Autodesk Fusion 360 part; units mm, degrees
sketch "草图1" plane through (0, 0, 0) normal (0, 1, 0) x (1, 0, 0)
  line L0 (0, 0) -> (95.2, 0)
  line L1 (95.2, 0) -> (95.2, 95.4)
  line L2 (95.2, 95.4) -> (0, 95.4)
  line L3 (0, 95.4) -> (0, 0)
  line L4 (-1.5, 96.9) -> (96.7, 96.9)
  line L5 (96.7, 96.9) -> (96.7, -1.5)
  line L6 (96.7, -1.5) -> (-1.5, -1.5)
  line L7 (-1.5, -1.5) -> (-1.5, 96.9)
  line L8 (-2.5, 97.9) -> (97.7, 97.9)
  line L9 (97.7, 97.9) -> (97.7, -2.5)
  line L10 (97.7, -2.5) -> (-2.5, -2.5)
  line L11 (-2.5, -2.5) -> (-2.5, 97.9)
  line L12 (-4.5, 100.9) -> (99.7, 100.9)
  line L13 (99.7, 100.9) -> (99.7, -5.5)
  line L14 (99.7, -5.5) -> (-4.5, -5.5)
  line L15 (-4.5, -5.5) -> (-4.5, 100.9)
  line L16 (99.7, 100.9) -> (79.7, 100.9)
  line L17 (79.7, 100.9) -> (79.7, 80.9)
  line L18 (79.7, 80.9) -> (99.7, 80.9)
  line L19 (99.7, 80.9) -> (99.7, 100.9)
  line L20 (79.7, 100.9) -> (99.7, 80.9)
  dimension "d1" = 95.2
  dimension "d2" = 95.4
  dimension "d3" = 1.5
  dimension "d4" = 1.5
  dimension "d5" = 1.5
  dimension "d6" = 1.5
  dimension "d7" = 1
  dimension "d8" = 1
  dimension "d9" = 1
  dimension "d10" = 1
  dimension "d11" = 3
  dimension "d12" = 2
  dimension "d13" = 2
  dimension "d14" = 3
  dimension "d21" = 20
  dimension "d22" = 20
extrude "拉伸1" add sketch "草图1" along normal blind 2 contours L0 L1 L2 L3 L17 L18 | L0 L1 L2 L3 L4 L5 L6 L7 L17 L18 | L1 L2 L17 L18 L20 | L1 L5 L18 L20 | L2 L4 L17 L20 | L1 L2 L20 | L1 L2 L4 L5 L20 | L4 L5 L6 L7 L8 L9 L10 L11 L17 L18 | L5 L9 L18 L20 | L4 L8 L17 L20 | L4 L5 L8 L9 L20
extrude "拉伸2" add sketch "草图1" along normal blind 22 contours L8 L9 L10 L11 L12 L13 L14 L15 L17 L18 | L9 L18 L20 | L8 L17 L20 | L8 L9 L12 L13 L16 L19 L20
fillet "圆角1" radius 5 4 edges at (-4.5, 11, 5.5) (99.7, 11, 5.5) (-4.5, 11, -100.9) (99.7, 11, -100.9)
extrude "拉伸3" [suppressed]
fillet "圆角2" [suppressed]
sketch "草图2" plane through (0, 2, 0) normal (0, 1, 0) x (-1, 0, 0)
  line L0 (-97.7, -97.9) -> (2.5, -97.9)
  line L1 (2.5, -97.9) -> (2.5, 2.5)
  line L2 (2.5, 2.5) -> (-97.7, 2.5)
  line L3 (-97.7, 2.5) -> (-97.7, -97.9)
  line L4 (2.5, 2.5) -> (2.5, -20)
  line L5 (2.5, -20) -> (-5.5, -20)
  line L6 (-5.5, -20) -> (-5.5, -22)
  line L7 (-5.5, -22) -> (2.5, -22)
  line L8 (2.5, -22) -> (2.5, -20)
  line L9 (-5.5, -20) -> (-3.5, -20)
  line L10 (-3.5, -20) -> (-3.5, 2.5)
  line L11 (-3.5, 2.5) -> (-5.5, 2.5)
  line L12 (-5.5, 2.5) -> (-5.5, -20)
  line L13 (-97.7, 2.5) -> (-91.7, 2.5)
  line L14 (-91.7, 2.5) -> (-91.7, -20)
  line L15 (-91.7, -20) -> (-97.7, -20)
  line L16 (-97.7, -20) -> (-97.7, 2.5)
  line L17 (-97.7, -20) -> (-89.7, -20)
  line L18 (-89.7, -20) -> (-89.7, -23)
  line L19 (-89.7, -23) -> (-97.7, -23)
  line L20 (-97.7, -23) -> (-97.7, -20)
  line L21 (-89.7, -20) -> (-91.7, -20)
  line L22 (-91.7, -20) -> (-91.7, 2.5)
  line L23 (-91.7, 2.5) -> (-89.7, 2.5)
  line L24 (-89.7, 2.5) -> (-89.7, -20)
  line L25 (-91.7, -97.9) -> (-91.7, -75.4)
  line L26 (-91.7, -97.9) -> (-97.7, -97.9)
  line L27 (-97.7, -97.9) -> (-97.7, -75.4)
  line L28 (-97.7, -75.4) -> (-91.7, -75.4)
  line L29 (2.5, -97.9) -> (2.5, -75.4)
  line L30 (-3.5, -75.4) -> (2.5, -75.4)
  line L31 (-3.5, -97.9) -> (-3.5, -75.4)
  line L32 (2.5, -97.9) -> (-3.5, -97.9)
  line L33 (2.5, -75.4) -> (-5.5, -75.4)
  line L34 (-5.5, -75.4) -> (-5.5, -73.4)
  line L35 (-5.5, -73.4) -> (2.5, -73.4)
  line L36 (2.5, -73.4) -> (2.5, -75.4)
  line L37 (-5.5, -75.4) -> (-3.5, -75.4)
  line L38 (-3.5, -75.4) -> (-3.5, -97.9)
  line L39 (-3.5, -97.9) -> (-5.5, -97.9)
  line L40 (-5.5, -97.9) -> (-5.5, -75.4)
  line L41 (-97.7, -75.4) -> (-89.7, -75.4)
  line L42 (-89.7, -75.4) -> (-89.7, -73.4)
  line L43 (-89.7, -73.4) -> (-97.7, -73.4)
  line L44 (-97.7, -73.4) -> (-97.7, -75.4)
  line L45 (-89.7, -75.4) -> (-91.7, -75.4)
  line L46 (-91.7, -75.4) -> (-91.7, -97.9)
  line L47 (-91.7, -97.9) -> (-89.7, -97.9)
  line L48 (-89.7, -97.9) -> (-89.7, -75.4)
  line L49 (-47.6, -97.9) -> (-47.6, -91.9)
  line L50 (-47.6, -91.9) -> (-36.35, -91.9)
  line L51 (-47.6, -91.9) -> (-58.85, -91.9)
  line L52 (-36.35, -91.9) -> (-58.85, -91.9)
  line L53 (-58.85, -91.9) -> (-58.85, -97.9)
  line L54 (-58.85, -97.9) -> (-36.35, -97.9)
  line L55 (-36.35, -97.9) -> (-36.35, -91.9)
  line L56 (-47.6, 2.5) -> (-36.35, 2.5)
  line L57 (-36.35, -3.5) -> (-36.35, 2.5)
  line L58 (-58.85, -3.5) -> (-36.35, -3.5)
  line L59 (-36.35, 2.5) -> (-58.85, 2.5)
  line L60 (-58.85, 2.5) -> (-58.85, -3.5)
  line L61 (-36.35, -97.9) -> (-34.35, -97.9)
  line L62 (-34.35, -97.9) -> (-34.35, -89.9)
  line L63 (-34.35, -89.9) -> (-36.35, -89.9)
  line L64 (-36.35, -89.9) -> (-36.35, -97.9)
  line L65 (-36.35, -89.9) -> (-58.85, -89.9)
  line L66 (-58.85, -89.9) -> (-58.85, -91.9)
  line L67 (-58.85, -91.9) -> (-36.35, -91.9)
  line L68 (-36.35, -91.9) -> (-36.35, -89.9)
  line L69 (-58.85, -89.9) -> (-60.85, -89.9)
  line L70 (-60.85, -89.9) -> (-60.85, -97.9)
  line L71 (-60.85, -97.9) -> (-58.85, -97.9)
  line L72 (-58.85, -97.9) -> (-58.85, -89.9)
  line L73 (-36.35, 2.5) -> (-34.35, 2.5)
  line L74 (-34.35, 2.5) -> (-34.35, -5.5)
  line L75 (-34.35, -5.5) -> (-36.35, -5.5)
  line L76 (-36.35, -5.5) -> (-36.35, 2.5)
  line L77 (-58.85, 2.5) -> (-60.85, 2.5)
  line L78 (-60.85, 2.5) -> (-60.85, -5.5)
  line L79 (-60.85, -5.5) -> (-58.85, -5.5)
  line L80 (-58.85, -5.5) -> (-58.85, 2.5)
  line L81 (-36.35, -5.5) -> (-58.85, -5.5)
  line L82 (-58.85, -5.5) -> (-58.85, -3.5)
  line L83 (-58.85, -3.5) -> (-36.35, -3.5)
  line L84 (-36.35, -3.5) -> (-36.35, -5.5)
  dimension "d27" = 22.5
  dimension "d28" = 8
  dimension "d29" = 2
  dimension "d32" = 6
  dimension "d33" = 22.5
  dimension "d34" = 8
  dimension "d35" = 3
  dimension "d38" = 77.9
  dimension "d39" = 0
  dimension "d42" = 94.2
  dimension "d43" = 0
  dimension "d44" = 8
  dimension "d45" = 2
  dimension "d46" = 8
  dimension "d47" = 2
  dimension "d50" = 6
  dimension "d51" = 11.25
  dimension "d52" = 11.25
  dimension "d55" = 0
  dimension "d56" = 94.4
  dimension "d57" = 2
  dimension "d58" = 8
  dimension "d59" = 2
  dimension "d60" = 8
  dimension "d61" = 2
  dimension "d62" = 8
  dimension "d63" = 2
  dimension "d64" = 8
extrude "拉伸4" [suppressed]
extrude "拉伸5" [suppressed]
extrude "拉伸6" [suppressed]
sketch "草图3" plane through (0, 2, 0) normal (0, 1, 0) x (-1, 0, 0)
  line L0 (2.5, 2.5) -> (-97.7, 2.5)
  line L1 (-97.7, 2.5) -> (-97.7, -97.9)
  line L2 (-97.7, -97.9) -> (2.5, -97.9)
  line L3 (2.5, -97.9) -> (2.5, 2.5)
  line L4 (2.5, 2.5) -> (-20, 2.5)
  line L5 (-20, 2.5) -> (-20, -4)
  line L6 (-20, -4) -> (2.5, -4)
  line L7 (2.5, -4) -> (2.5, 2.5)
  line L8 (2.5, -4) -> (-20, -4)
  line L9 (-20, -4) -> (-20, -6)
  line L10 (-20, -6) -> (2.5, -6)
  line L11 (2.5, -6) -> (2.5, -4)
  line L12 (-20, -6) -> (-22, -6)
  line L13 (-22, -6) -> (-22, 2.5)
  line L14 (-22, 2.5) -> (-20, 2.5)
  line L15 (-20, 2.5) -> (-20, -6)
  line L16 (-20, -91.4) -> (-20, -97.9)
  line L17 (-20, -97.9) -> (2.5, -97.9)
  line L18 (2.5, -97.9) -> (2.5, -91.4)
  line L19 (2.5, -91.4) -> (-20, -91.4)
  line L20 (2.5, -97.9) -> (-20, -97.9)
  line L21 (2.5, -91.4) -> (-20, -91.4)
  line L22 (-20, -91.4) -> (-20, -89.4)
  line L23 (-20, -89.4) -> (2.5, -89.4)
  line L24 (2.5, -89.4) -> (2.5, -91.4)
  line L25 (-20, -89.4) -> (-22, -89.4)
  line L26 (-22, -89.4) -> (-22, -97.9407)
  line L27 (-22, -97.9407) -> (-20, -97.9407)
  line L28 (-20, -97.9407) -> (-20, -89.4)
  line L29 (2.5, -47.7) -> (-4, -47.7)
  line L30 (-4, -47.7) -> (-4, -58.95)
  line L31 (-4, -58.95) -> (2.5, -58.95)
  line L32 (2.5, -58.95) -> (2.5, -47.7)
  line L33 (-4, -47.7) -> (2.5, -47.7)
  line L34 (2.5, -47.7) -> (2.5, -36.45)
  line L35 (2.5, -36.45) -> (-4, -36.45)
  line L36 (-4, -36.45) -> (-4, -47.7)
  line L37 (-97.7, -36.45) -> (-97.7, -47.7)
  line L38 (-91.2, -47.7) -> (-91.2, -36.45)
  line L39 (-97.7, -47.7) -> (-97.7, -58.95)
  line L40 (-91.2, -58.95) -> (-91.2, -47.7)
  line L41 (-91.2, -36.45) -> (-97.7, -36.45)
  line L42 (-91.2, -47.7) -> (-97.7, -47.7)
  line L43 (-97.7, -47.7) -> (-91.2, -47.7)
  line L44 (-97.7, -58.95) -> (-91.2, -58.95)
  line L45 (2.5, -36.45) -> (-6, -36.45)
  line L46 (-6, -36.45) -> (-6, -34.45)
  line L47 (-6, -34.45) -> (2.5, -34.45)
  line L48 (2.5, -34.45) -> (2.5, -36.45)
  line L49 (-4, -58.95) -> (-6, -58.95)
  line L50 (-6, -58.95) -> (-6, -36.45)
  line L51 (-6, -36.45) -> (-4, -36.45)
  line L52 (-4, -36.45) -> (-4, -58.95)
  line L53 (-6, -58.95) -> (2.5, -58.95)
  line L54 (2.5, -58.95) -> (2.5, -60.95)
  line L55 (2.5, -60.95) -> (-6, -60.95)
  line L56 (-6, -60.95) -> (-6, -58.95)
  line L57 (-97.7, -36.45) -> (-89.2, -36.45)
  line L58 (-89.2, -36.45) -> (-89.2, -34.45)
  line L59 (-89.2, -34.45) -> (-97.7, -34.45)
  line L60 (-97.7, -34.45) -> (-97.7, -36.45)
  line L61 (-89.2, -36.45) -> (-91.2, -36.45)
  line L62 (-91.2, -36.45) -> (-91.2, -58.95)
  line L63 (-91.2, -58.95) -> (-89.2, -58.95)
  line L64 (-89.2, -58.95) -> (-89.2, -36.45)
  line L65 (-89.2, -58.95) -> (-97.7, -58.95)
  line L66 (-97.7, -58.95) -> (-97.7, -60.95)
  line L67 (-97.7, -60.95) -> (-89.2, -60.95)
  line L68 (-89.2, -60.95) -> (-89.2, -58.95)
  line L69 (-101, -101) -> (-85, -101)
  line L70 (-85, -101) -> (-85, -85)
  line L71 (-85, -85) -> (-101, -85)
  line L72 (-101, -85) -> (-101, -101)
  line L73 (-85, -97.9) -> (-83, -97.9)
  line L74 (-83, -97.9) -> (-83, -89.4)
  line L75 (-83, -89.4) -> (-85, -89.4)
  line L76 (-85, -89.4) -> (-85, -97.9)
  line L77 (-83, -97.9) -> (-60.5, -97.9)
  line L78 (-60.5, -97.9) -> (-60.5, -91.4)
  line L79 (-60.5, -91.4) -> (-83, -91.4)
  line L80 (-83, -91.4) -> (-83, -97.9)
  line L81 (-83, -89.4) -> (-60.5, -89.4)
  line L82 (-60.5, -89.4) -> (-60.5, -91.4)
  line L83 (-60.5, -91.4) -> (-83, -91.4)
  line L84 (-83, -91.4) -> (-83, -89.4)
  line L85 (-60.5, -89.4) -> (-58.5, -89.4)
  line L86 (-58.5, -89.4) -> (-58.5, -97.9)
  line L87 (-58.5, -97.9) -> (-60.5, -97.9)
  line L88 (-60.5, -97.9) -> (-60.5, -89.4)
  line L89 (-60.5, 2.5) -> (-83, 2.5)
  line L90 (-60.5, 2.5) -> (-83, 2.5)
  line L91 (-83, -4) -> (-60.5, -4)
  line L92 (-60.5, -4) -> (-60.5, 2.5)
  line L93 (-83, 2.5) -> (-83, -4)
  line L94 (-60.5, 2.5) -> (-58.5, 2.5)
  line L95 (-58.5, 2.5) -> (-58.5, -6)
  line L96 (-58.5, -6) -> (-60.5, -6)
  line L97 (-60.5, -6) -> (-60.5, 2.5)
  line L98 (-60.5, -6) -> (-83, -6)
  line L99 (-83, -6) -> (-83, -4)
  line L100 (-83, -4) -> (-60.5, -4)
  line L101 (-60.5, -4) -> (-60.5, -6)
  line L102 (-83, -6) -> (-85, -6)
  line L103 (-85, -6) -> (-85, 2.5)
  line L104 (-85, 2.5) -> (-83, 2.5)
  line L105 (-83, 2.5) -> (-83, -6)
  point P0 (-20, -91.4)
  point P1 (2.5, -91.4)
  point P2 (0, -93.9)
  point P3 (-60.5, -4)
  dimension "d67" = 22.5
  dimension "d68" = 6.5
  dimension "d69" = 22.5
  dimension "d70" = 2
  dimension "d79" = 2
  dimension "d80" = 2
  dimension "d84" = 6.5
  dimension "d85" = 11.25
  dimension "d86" = 11.25
  dimension "d89" = -93.7
  dimension "d90" = 0
  dimension "d91" = 8.5
  dimension "d92" = 2
  dimension "d93" = 2
  dimension "d94" = 8.5
  dimension "d95" = 2
  dimension "d96" = 2
  dimension "d101" = 2
  dimension "d102" = 8.5
  dimension "d103" = 22.5
  dimension "d104" = 6.5
  dimension "d105" = 2
  dimension "d108" = -93.9
  dimension "d109" = 0
  dimension "d110" = 2
  dimension "d111" = 8.5
  dimension "d112" = 2
extrude "拉伸8" cut sketch "草图3" along normal blind 24 contours L1 L2 L69 L70 L71 L72
extrude "拉伸9" add sketch "草图3" along normal blind 4 contours L0 L5 L9 L12 L13 L14 L15 | L3 L6 L8 L9 L10 L11 L15 | L0 L92 L94 L95 L96 L97 L101 | L3 L35 L45 L46 L47 L48 L51 | L0 L93 L99 L102 L103 L104 L105 | L91 L97 L98 L99 L100 L101 L105 | L30 L36 L45 L49 L50 L51 L52 L53 | L3 L31 L49 L53 L54 L55 L56 | L1 L41 L57 L58 L59 L60 L61 | L3 L19 L21 L22 L23 L24 L28 | L2 L16 L22 L25 L26 L28 | L38 L40 L57 L61 L62 L63 L64 L65 | L1 L44 L63 L65 L66 L67 L68 | L2 L78 L82 L85 L86 L87 L88 | L2 L70 L73 L74 L75 L76 L80 L84 | L74 L79 L81 L82 L83 L84 L88
Could you check a few things on this model? Use its own coordinates, in mm. A direction names the side the tool comes from. Round coordinates to 2 decimals unless told otherwise and drop trailing zeros. Write each loop counter-clockwise with the first axis right and the second up, starting at its lowest first coordinate (ties: lowest second). Pieces come first, ordered by that corner, then holes. Notation, with made-up numbers: M 56.5,6 L 63.5,6 A27 cw 63.5,37 Z; hole C -0.75,-9 d5. An arc over 180 degrees is marked long. Answer in a Markdown table with one row per item. Add a question column.
Q1. Will these pins go through, and if not, where does the flat tip stop? pin 1 Ø12 at (x, z) = (85, -32) entering from +Y; pin 2 Ø5 at (x, z) = (81.5, -75.5) entering from +Y; pin 3 Ø1.2 at (y, z) = (5, -92.5) entering from +X.
Q2. Imagine slicing it at D-D (z = -38.5). Please give me the cut outline in (x, y), then the cut area to 3 significant figures.
Q3. If I drill on line 1 (Z direction, x = 7, y = 3); line 2 (Z direction, x = 5, y = 4); line 3 (X direction, y = 18, z = -84), over which ranges is the centre line in solid material (lowest first)? Write a range as from..to.
Q4. Imagine slicing it at A-A (z = -25). Please give me the cut outline in (x, y).
Q5. Imagine slicing it at C-C (y = 17.25). Please give me the cut outline in (x, z).
Q6. On a 3-axis mill with a long thin cutter (end or side, diameter ignored), from which of +Z, -Z, +X, -X, +Y, -Y can I reach the whole of each face in a straight line? I mean faces 4 (the flat face through (72, 4, -89.4)), 5 (the flat face through (5, 6, -48)), 6 (the cylindrical face through (98.27, 1.01, -99.4)), 7 (the flat face through (91, 6, -48)). Say none if no direction works.
Q7. Imagine slicing it at B-B (x = 68.5). Please give me the cut outline in (y, z), then the cut area to 3 significant figures.
Q8. If we mould it in two halves opening along X, with no side actions, what happens to faces 1 (the flat face through (99.7, 11, -48)), 2 (the flat face through (47, 11, -100.9)), 3 (the flat face through (9, 2, -1))? For each: +X half, -X half, draft (parallel to the pull), parting line (faces both ways), or undercut.
Values:
| question | item | result |
|---|---|---|
| 1 | pin 1 | y = 6 |
| 1 | pin 2 | y = 2 |
| 1 | pin 3 | x = 85 |
| 2 | outline | M -4.5,0 L 99.7,0 L 99.7,22 L 97.7,22 L 97.7,2 L 91.2,2 L 91.2,6 L 89.2,6 L 89.2,2 L 6,2 L 6,6 L 4,6 L 4,2 L -2.5,2 L -2.5,22 L -4.5,22 Z |
| 2 | area | 304 mm^2 |
| 3 | line 1 | -100.9..-97.9, -91.4..-89.4, -6..-4, 2.5..5.5 |
| 3 | line 2 | -100.9..-97.9, -91.4..-89.4, -60.95..-34.45, -6..-4, 2.5..5.5 |
| 3 | line 3 | -4.5..-2.5, 97.7..99.7 |
| 4 | outline | M -4.5,0 L 99.7,0 L 99.7,22 L 97.7,22 L 97.7,2 L -2.5,2 L -2.5,22 L -4.5,22 Z |
| 5 | outline | M -4.5,-95.9 A5 ccw 0.5,-100.9 L 85,-100.9 L 85,-97.9 L -2.5,-97.9 L -2.5,2.5 L 97.7,2.5 L 97.7,-85 L 99.7,-85 L 99.7,0.5 A5 ccw 94.7,5.5 L 0.5,5.5 A5 ccw -4.5,0.5 Z |
| 6 | face 4 | +X, +Y |
| 6 | face 5 | +Y |
| 6 | face 6 | -Z, +X, +Y, -Y |
| 6 | face 7 | -Z, +Y |
| 7 | outline | M 0,-100.9 L 22,-100.9 L 22,-97.9 L 2,-97.9 L 2,-91.4 L 6,-91.4 L 6,-89.4 L 2,-89.4 L 2,-6 L 6,-6 L 6,-4 L 2,-4 L 2,2.5 L 22,2.5 L 22,5.5 L 0,5.5 Z |
| 7 | area | 349 mm^2 |
| 8 | face 1 | +X half |
| 8 | face 2 | draft |
| 8 | face 3 | undercut |
